Check sheet for the modelled part. Datum: model origin and axes. Units: mm. A direction names the side the tool comes from. Coordinates: 2 decimals unless noted, no trailing zeros. Write each loop counter-clockwise with the first axis right and the second up, starting at its lowest first coordinate (ties: lowest second). Pieces come first, ordered by that corner, then holes. Notation, with made-up numbers: (-7, 50.5) - (15, 50.5) arc R21 cw to (15, 87.5) - close; hole circle Ø4 at (-3, 1). An arc over 180 degrees is marked (long way). Write each question's results on one line, items separated by ' | '.
from build123d import *

# Parameters (mm, degrees)
SKETCH1_R           = 5
SKETCH1_R_2         = 3
BOSS_EXTRUDE1_DEPTH = 0.5
CUT_EXTRUDE2_DEPTH  = 0.5
CUT_EXTRUDE3_DEPTH  = 0.5
CUT_EXTRUDE5_DEPTH  = 0.5


with BuildPart() as part:
    # Sketch1 → Boss-Extrude1 (new body)
    with BuildSketch(Plane(origin=(0, 0, 0), x_dir=(1, 0, 0), z_dir=(0, 1, 0))):
        Circle(SKETCH1_R)
        Circle(SKETCH1_R_2, mode=Mode.SUBTRACT)
    extrude(amount=BOSS_EXTRUDE1_DEPTH)

    # Sketch1<4> → Cut-Extrude2 (cut)
    with BuildSketch(Plane(origin=(0, 0, 0), x_dir=(1, 0, 0), z_dir=(0, 1, 0))):
        with BuildLine():
            ThreePointArc((-3.744681424, 2.694339182), (-3.662355303, 1.691396556), (-3.06721905, 0.879926074))
            ThreePointArc((-3.06721905, 0.879926074), (-3.041225351, 0.669392639), (-3.251758787, 0.64339894))
            ThreePointArc((-3.251758787, 0.64339894), (-3.943403621, 1.586459229), (-4.039079925, 2.7520412))
            ThreePointArc((-4.039079925, 2.7520412), (-3.863029666, 2.870389441), (-3.744681424, 2.694339182))
        make_face()
    extrude(amount=CUT_EXTRUDE2_DEPTH, mode=Mode.SUBTRACT)

    # Sketch1<6> → Cut-Extrude3 (cut)
    with BuildSketch(Plane(origin=(0, 0, 0), x_dir=(1, 0, 0), z_dir=(0, 1, 0))):
        with BuildLine():
            ThreePointArc((2.7520412, 4.039079925), (1.586459229, 3.943403621), (0.64339894, 3.251758787))
            ThreePointArc((0.64339894, 3.251758787), (0.669392639, 3.041225351), (0.879926074, 3.06721905))
            ThreePointArc((0.879926074, 3.06721905), (1.691396556, 3.662355303), (2.694339182, 3.744681424))
            ThreePointArc((2.694339182, 3.744681424), (2.870389441, 3.863029666), (2.7520412, 4.039079925))
        make_face()
        with BuildLine():
            ThreePointArc((-1.895819652, 4.20570689), (-2.325994452, 3.295970036), (-2.216326579, 2.295647859))
            ThreePointArc((-2.216326579, 2.295647859), (-2.299082093, 2.100323706), (-2.494406247, 2.18307922))
            ThreePointArc((-2.494406247, 2.18307922), (-2.621858099, 3.345615805), (-2.121925223, 4.402877554))
            ThreePointArc((-2.121925223, 4.402877554), (-1.910287106, 4.417345007), (-1.895819652, 4.20570689))
        make_face()
        with BuildLine():
            ThreePointArc((0.461025466, 4.590158833), (-0.366385266, 4.017391008), (-0.771571191, 3.096252653))
            ThreePointArc((-0.771571191, 3.096252653), (-0.940901645, 2.968474732), (-1.068679567, 3.137805186))
            ThreePointArc((-1.068679567, 3.137805186), (-0.597787817, 4.208317328), (0.363797629, 4.873966423))
            ThreePointArc((0.363797629, 4.873966423), (0.554315342, 4.780676547), (0.461025466, 4.590158833))
        make_face()
    extrude(amount=CUT_EXTRUDE3_DEPTH, mode=Mode.SUBTRACT)

    # Sketch1<7> → Cut-Extrude5 (cut)
    with BuildSketch(Plane(origin=(0, 0, 0), x_dir=(1, 0, 0), z_dir=(0, 1, 0))):
        with BuildLine():
            ThreePointArc((4.20570689, 1.895819652), (3.295970036, 2.325994452), (2.295647859, 2.216326579))
            ThreePointArc((2.295647859, 2.216326579), (2.100323706, 2.299082093), (2.18307922, 2.494406247))
            ThreePointArc((2.18307922, 2.494406247), (3.345615805, 2.621858099), (4.402877554, 2.121925223))
            ThreePointArc((4.402877554, 2.121925223), (4.417345007, 1.910287106), (4.20570689, 1.895819652))
        make_face()
        with BuildLine():
            ThreePointArc((4.590158833, -0.461025466), (4.017391008, 0.366385266), (3.096252653, 0.771571191))
            ThreePointArc((3.096252653, 0.771571191), (2.968474732, 0.940901645), (3.137805186, 1.068679567))
            ThreePointArc((3.137805186, 1.068679567), (4.208317328, 0.597787817), (4.873966423, -0.363797629))
            ThreePointArc((4.873966423, -0.363797629), (4.780676547, -0.554315342), (4.590158833, -0.461025466))
        make_face()
        with BuildLine():
            ThreePointArc((3.744681424, -2.694339182), (3.662355303, -1.691396556), (3.06721905, -0.879926074))
            ThreePointArc((3.06721905, -0.879926074), (3.041225351, -0.669392639), (3.251758787, -0.64339894))
            ThreePointArc((3.251758787, -0.64339894), (3.943403621, -1.586459229), (4.039079925, -2.7520412))
            ThreePointArc((4.039079925, -2.7520412), (3.863029666, -2.870389441), (3.744681424, -2.694339182))
        make_face()
        with BuildLine():
            ThreePointArc((1.895819652, -4.20570689), (2.325994452, -3.295970036), (2.216326579, -2.295647859))
            ThreePointArc((2.216326579, -2.295647859), (2.299082093, -2.100323706), (2.494406247, -2.18307922))
            ThreePointArc((2.494406247, -2.18307922), (2.621858099, -3.345615805), (2.121925223, -4.402877554))
            ThreePointArc((2.121925223, -4.402877554), (1.910287106, -4.417345007), (1.895819652, -4.20570689))
        make_face()
        with BuildLine():
            ThreePointArc((-0.461025466, -4.590158833), (0.366385266, -4.017391008), (0.771571191, -3.096252653))
            ThreePointArc((0.771571191, -3.096252653), (0.940901645, -2.968474732), (1.068679567, -3.137805186))
            ThreePointArc((1.068679567, -3.137805186), (0.597787817, -4.208317328), (-0.363797629, -4.873966423))
            ThreePointArc((-0.363797629, -4.873966423), (-0.554315342, -4.780676547), (-0.461025466, -4.590158833))
        make_face()
        with BuildLine():
            ThreePointArc((-2.694339182, -3.744681424), (-1.691396556, -3.662355303), (-0.879926074, -3.06721905))
            ThreePointArc((-0.879926074, -3.06721905), (-0.669392639, -3.041225351), (-0.64339894, -3.251758787))
            ThreePointArc((-0.64339894, -3.251758787), (-1.586459229, -3.943403621), (-2.7520412, -4.039079925))
            ThreePointArc((-2.7520412, -4.039079925), (-2.870389441, -3.863029666), (-2.694339182, -3.744681424))
        make_face()
        with BuildLine():
            ThreePointArc((-4.20570689, -1.895819652), (-3.295970036, -2.325994452), (-2.295647859, -2.216326579))
            ThreePointArc((-2.295647859, -2.216326579), (-2.100323706, -2.299082093), (-2.18307922, -2.494406247))
            ThreePointArc((-2.18307922, -2.494406247), (-3.345615805, -2.621858099), (-4.402877554, -2.121925223))
            ThreePointArc((-4.402877554, -2.121925223), (-4.417345007, -1.910287106), (-4.20570689, -1.895819652))
        make_face()
        with BuildLine():
            ThreePointArc((-4.590158833, 0.461025466), (-4.017391008, -0.366385266), (-3.096252653, -0.771571191))
            ThreePointArc((-3.096252653, -0.771571191), (-2.968474732, -0.940901645), (-3.137805186, -1.068679567))
            ThreePointArc((-3.137805186, -1.068679567), (-4.208317328, -0.597787817), (-4.873966423, 0.363797629))
            ThreePointArc((-4.873966423, 0.363797629), (-4.780676547, 0.554315342), (-4.590158833, 0.461025466))
        make_face()
    extrude(amount=CUT_EXTRUDE5_DEPTH, mode=Mode.SUBTRACT)


solid = part.part
1. Access from +Z, -Z, +X, -X, +Y, -Y to the whole of each face (thin tool, end or side, straight path). Record for faces 1 (the cylindrical face through (0.608, 0.246, 4.195)), 2 (the flat face through (-0.1, 0, 3.3)).
Values follow:
face 1: +Y, -Y | face 2: +Z, -Z, +X, -X, -Y
2. Draft check along X on faces 3 (the cylindrical face through (4.195, 0.246, -0.608)), 4 (the flat face through (-0.1, 0.5, 3.3)), 5 (the cylindrical face through (-1.08, 0.25, 4.88)). Enter one of: pulls with the +X half, pulls with the -X half, needs draft (parallel to the pull), parting line crosses it, or undercut.
Values follow:
face 3: undercut | face 4: needs draft | face 5: parting line crosses it
3. Sectioned sample at D-D (y = 0.25). Give the number of separate pieces and of enclosed holes in the cut face, then the cut area to 3 significant figures.
Values follow:
separate pieces: 1 | enclosed holes: 13 | area: 41.5 mm^2
4. Sectioned sample at A-A (x = -0.25). Record the cut outline in (y, z), then the cut area to 3 significant figures.
Values follow:
outline: (0, -4.99) - (0.5, -4.99) - (0.5, -4.54) - (0, -4.54) - close; (0, -4.15) - (0.5, -4.15) - (0.5, -2.99) - (0, -2.99) - close; (0, 2.99) - (0.5, 2.99) - (0.5, 4.5) - (0, 4.5) - close; (0, 4.83) - (0.5, 4.83) - (0.5, 4.99) - (0, 4.99) - close | area: 1.64 mm^2
5. Sectioned sample at B-B (z = -1.5). Record the cut outline in (x, y), then the cut area to 3 significant figures.
Values follow:
outline: (-4.77, 0) - (-3.91, 0) - (-3.91, 0.5) - (-4.77, 0.5) - close; (-3.58, 0) - (-2.6, 0) - (-2.6, 0.5) - (-3.58, 0.5) - close; (2.6, 0) - (4.77, 0) - (4.77, 0.5) - (2.6, 0.5) - close | area: 2.01 mm^2
6. Sectioned sample at C-C (z = 0). Record the cut outline in (x, y), then the cut area to 3 significant figures.
Values follow:
outline: (-5, 0) - (-4.71, 0) - (-4.71, 0.5) - (-5, 0.5) - close; (-4.36, 0) - (-3, 0) - (-3, 0.5) - (-4.36, 0.5) - close; (3, 0) - (4.36, 0) - (4.36, 0.5) - (3, 0.5) - close; (4.71, 0) - (5, 0) - (5, 0.5) - (4.71, 0.5) - close | area: 1.65 mm^2
7. Material ranges on L1, parallel to X at y = 0.4, z = 0; L2, parallel to X at y = 0.35, z = 0.25, recorded low to high. Write a range as [from, to].
Values follow:
L1: x = [-5, -4.71], [-4.36, -3], [3, 4.36], [4.71, 5] | L2: x = [-4.99, -4.54], [-4.15, -2.99], [2.99, 4.5], [4.83, 4.99]
8. Go/stop test with a flat-tipped pin: pin 1 (5.5 mm diameter, centred on x = 0, z = 0, fed in from -Y) (3 decimals). Record where the tip stops, or that it passes through.
Values follow:
pin 1: passes through
